Autodesk Inventor part; units mm, degrees
ref_plane "YZ Plane" through (0, 0, 0) normal (1, 0, 0) x (0, 1, 0)
ref_plane "XZ Plane" through (0, 0, 0) normal (0, 1, 0) x (-1, 0, 0)
ref_plane "XY Plane" through (0, 0, 0) normal (0, 0, 1) x (1, 0, 0)
sketch "Sketch1" plane through (0, 0, 0) normal (0, 0, 1) x (1, 0, 0)
  circle A0 centre (-45.2437, 35.97) radius 1.27
  circle A1 centre (10.6363, 18.2563) radius 3.175
  line L0 (-71.7503, -2.6941) -> (-71.7503, 45.5566)
  line L1 (69.7183, -2.6941) -> (-71.7503, -2.6941)
  line L2 (69.7183, 45.5566) -> (69.7183, -2.6941)
  line L3 (-71.7503, 45.5566) -> (69.7183, 45.5566)
  line L4 (99.568, 75.4063) -> (99.568, -32.5437)
  line L5 (99.568, -32.5437) -> (-101.6, -32.5438)
  line L6 (-101.6, -32.5438) -> (-101.6, 75.4062)
  line L7 (-101.6, 75.4062) -> (99.568, 75.4063)
  line L8 (18.8383, 62.7063) -> (74.667, 62.7063)
  line L9 (74.667, 62.7063) -> (74.667, -26.1937)
  line L10 (74.667, -26.1937) -> (18.8383, -26.1937)
  line L11 (18.8383, -26.1937) -> (18.8383, 62.7063)
  line L12 (99.568, 21.4313) -> (-101.6, 21.4312) construction
  line L13 (8.6043, 3.175) -> (8.6043, 21.4313) construction
  point P0 (0, 0)
  dimension "d2" = 201.168
  dimension "d3" = 107.95
  dimension "d4" = 107.95
  dimension "d5" = 90
  dimension "d6" = 201.168
  dimension "d7" = 12.7
  dimension "d8" = 88.9
extrude "Extrusion1" add sketch "Sketch1" along normal blind 6.35 contours L0 L3 L11 L1 | L4 L5 L6 L7
sketch "Sketch2" plane through (0, 0, 0) normal (0, 0, -1) x (-1, 0, 0)
  line L0 (101.6, -32.5438) -> (101.6, 75.4062)
  line L1 (107.95, 65.692) -> (107.95, 61.9836)
  line L2 (107.95, 11.4304) -> (107.95, 7.722)
  line L3 (101.6, 7.722) -> (107.95, 7.722) construction
  line L4 (101.6, 11.4304) -> (107.95, 11.4304) construction
  line L5 (101.6, 61.9836) -> (107.95, 61.9836) construction
  line L6 (101.6, 65.4439) -> (107.95, 65.4439) construction
  line L7 (101.6, 7.722) -> (88.9, 7.722)
  line L8 (88.9, 7.722) -> (88.9, 11.4304)
  line L9 (88.9, 11.4304) -> (101.6, 11.4304)
  line L10 (101.6, 11.4304) -> (101.6, 7.722)
  line L11 (101.6, 61.9836) -> (88.9, 61.9836)
  line L12 (88.9, 61.9836) -> (88.9, 65.692)
  line L13 (88.9, 65.692) -> (101.6, 65.692)
  line L14 (101.6, 65.692) -> (101.6, 61.9836)
  line L15 (92.456, 5.6392) -> (95.25, 5.6392)
  line L16 (95.25, 5.6392) -> (95.25, 13.5132)
  line L17 (95.25, 13.5132) -> (92.456, 13.5132)
  line L18 (92.456, 13.5132) -> (92.456, 5.6392)
  line L19 (92.456, 59.9008) -> (95.25, 59.9008)
  line L20 (95.25, 59.9008) -> (95.25, 67.7748)
  line L21 (95.25, 67.7748) -> (92.456, 67.7748)
  line L22 (92.456, 67.7748) -> (92.456, 59.9008)
  point P0 (0, 0)
  dimension "d9" = 12.7
  dimension "d10" = 2.794
  dimension "d11" = 7.874
  dimension "d12" = 7.874
  dimension "d13" = 2.794
  dimension "d14" = 2.0828
  dimension "d16" = 2.0828
  dimension "d17" = 2.0828
  dimension "d18" = 6.35
  dimension "d19" = 6.35
extrude "Extrusion2" cut sketch "Sketch2" against normal through all
ref_plane "Work Plane1" through (-1.016, -32.5437, 0) normal (-1, 0, 0) x (0, 0, 1)
mirror "Mirror1" about plane through (-1.016, -32.5437, 0) normal (-1, 0, 0) of "Extrusion2"
equation "\"d4\" = d3"
equation "\"d6\" = d2"
equation "\"d13\" = d10"
equation "\"d14\" = d16"
equation "\"d17\" = d14"
equation "\"d19\" = d18"
properties part number "projectorMountingBase" material "Steel, Wrought"
Could you check a few things on this model? Use its own coordinates, in mm. A direction names the side the tool comes from. Give positions to 0.01 mm unless a question says otherwise; leave off trailing zeros. Write each loop counter-clockwise with the first axis right and the second up, starting at its lowest first coordinate (ties: lowest second). Pieces come first, ordered by that corner, then holes. Notation, with made-up numbers: (27, -1.75) - (79, -1.75) arc R24 ccw to (79, 31.25) - close; hole circle Ø5 at (88.25, 36.5). An arc over 180 degrees is marked (long way). Use CSV: the item, a comma, the result in double quotes. Start each with the question number.
Item 1: I want a section at A-A, the plane y = 30.5. Please give me the cut outline in (x, z), then the cut area to 3 significant figures.
Item 2: For faces 1 (the face through (-101.6, 36, 3)), 2 (the face through (96, 11.43, 3)), 3 (the face through (-91, 61.984, 3)), 4 (the face through (46, 62.706, 3)), which set-ups out of +Z, -Z, +X, -X, +Y, -Y let a thin tool reach every point of the face, with its end or its side?
Item 3: I want a section at B-B, the plane x = 35.5. Please give me the cut outline in (y, z).
Item 4: I'm going to push a flat-ended pin straight in: pin 1 (1.1 mm diameter, centred on y = 10, z = 3, fed in from +X). Where does the tip first touch, or does it pass through?
Item 5: I want a section at C-C, the plane z = 4.25. Give the number of separate pieces and of enclosed holes in the cut face, then the cut area to 3 significant figures.
Item 6: If we mould it in two halves opening along Y, with no side actions, what happens to faces 5 (the face through (-88.9, 10, 3)), 6 (the face through (99.568, -12, 3)), 7 (the face through (-88.9, 64, 3))? For each: pulls with the +Y half, pulls with the -Y half, needs draft (parallel to the pull), parting line crosses it, or undercut.
Item 7: If I drill on line 1 along X through (y, z) = (17, 0.75); line 2 along X through (y, z) = (26, 0.5); line 3 along Y through (x, z) = (69, 5.5), over which ranges is the centre line in solid material (lowest first)?
Findings:
1,outline,"(-101.6, 0) - (18.84, 0) - (18.84, 6.35) - (-101.6, 6.35) - close; (74.67, 0) - (99.57, 0) - (99.57, 6.35) - (74.67, 6.35) - close"
1,area,"923 mm2"
2,face 1,"+Z, -Z, -X, +Y, -Y"
2,face 2,"+Z, -Z, +X"
2,face 3,"+Z, -Z, -X"
2,face 4,"+Z, -Z"
3,outline,"(-32.54, 0) - (-26.19, 0) - (-26.19, 6.35) - (-32.54, 6.35) - close; (62.71, 0) - (75.41, 0) - (75.41, 6.35) - (62.71, 6.35) - close"
4,pin 1,"stops at x = 86.87"
5,separate pieces,"1"
5,enclosed holes,"3"
5,area,"16,500 mm2"
6,face 5,"undercut"
6,face 6,"needs draft"
6,face 7,"undercut"
7,line 1,"x = -101.6 to 7.72, 13.55 to 18.84, 74.67 to 99.57"
7,line 2,"x = -101.6 to 18.84, 74.67 to 99.57"
7,line 3,"y = -32.54 to -26.19, 62.71 to 75.41"
